Here's how the part is built. I have some questions about the finished solid (model axes, mm). Face numbers are marked on the shaded views. A direction names the side the tool comes from. Give positions to 0.01 mm unless a question says otherwise; leave off trailing zeros. Loops run counter-clockwise (first coordinate to the right, second up) from the corner with the lowest first, then second, coordinate; pieces in that order, holes last.
Q1. I need wall thicknesses on line 1 (Z direction, x = -1.5, y = -5); line 2 (Z direction, x = -19.5, y = 16); line 3 (X direction, y = 0.5, z = -30). Which ranges of each line are inside material? Lowest first, please.
Q2. Will these pins go through, and if not, where does the flat tip stop? P1, Ø4, axis at x = 12.5, y = 19, coming from the -Z side; P2, Ø12, axis at x = -9, z = 3.5, coming from the +Y side; P3, Ø2, axis at y = -3.5, z = -57, coming from the -X side.
Q3. If we section it at C-C (z = 54): Please give me the cut outline in (x, y), plus the area to 3 significant figures.
Q4. If we section it at D-D (x = -11): Please give me the cut outline in (y, z), plus the area to 3 significant figures.
Q5. If we section it at A-A (x = 0): Please give me the cut outline in (y, z).
Q6. For the marked faces 1, 2 and 3, which set-ups out of +Z, -Z, +X, -X, +Y, -Y let a thin tool reach every point of the face, with its end or its side?
from build123d import *

# Parameters (mm, degrees)
F0_R     = 5.085856
F1_DEPTH = 75
F0_R_2   = 14.586224
F2_DEPTH = 35
F0_R_3   = 25.413883
F3_DEPTH = 15


with BuildPart() as f1:
    # F0 (on Top) → F1 (new body, symmetric)
    with BuildSketch(Plane.XY):
        Circle(F0_R)
    extrude(amount=F1_DEPTH, both=True)

    # F0 (on Top) → F2 (join, symmetric)
    with BuildSketch(Plane.XY):
        Circle(F0_R_2)
        Circle(F0_R, mode=Mode.SUBTRACT)
    extrude(amount=F2_DEPTH, both=True)

    # F0 (on Top) → F3 (join, symmetric)
    with BuildSketch(Plane.XY):
        Circle(F0_R_3)
        Circle(F0_R_2, mode=Mode.SUBTRACT)
    extrude(amount=F3_DEPTH, both=True)


solid = f1.part
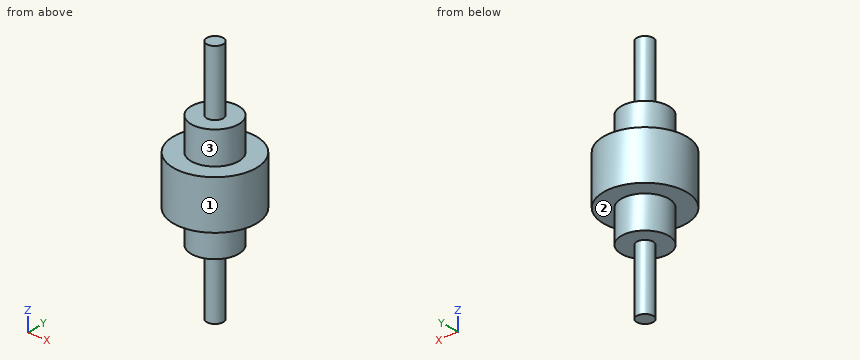
Check sheet entries:
1. line 1: z = -35 to 35
1. line 2: z = -15 to 15
1. line 3: x = -14.58 to 14.58
2. P1: stops at z = -15
2. P2: stops at y = 25.24
2. P3: stops at x = -4.43
3. outline: circle Ø10.17 at (0, 0)
3. area: 81.3 mm2
4. outline: (-22.91, -15) - (-9.58, -15) - (-9.58, -35) - (9.58, -35) - (9.58, -15) - (22.91, -15) - (22.91, 15) - (9.58, 15) - (9.58, 35) - (-9.58, 35) - (-9.58, 15) - (-22.91, 15) - close
4. area: 2,140 mm2
5. outline: (-25.41, -15) - (-14.59, -15) - (-14.59, -35) - (-5.09, -35) - (-5.09, -75) - (5.09, -75) - (5.09, -35) - (14.59, -35) - (14.59, -15) - (25.41, -15) - (25.41, 15) - (14.59, 15) - (14.59, 35) - (5.09, 35) - (5.09, 75) - (-5.09, 75) - (-5.09, 35) - (-14.59, 35) - (-14.59, 15) - (-25.41, 15) - close
6. face 1: +Z, -Z
6. face 2: -Z
6. face 3: +Z
